```python
from build123d import *

# Parameters (mm, degrees)
F0_W     = 2133.6
F0_H     = 609.6
F1_DEPTH = 762
F3_DEPTH = 15240
F2_W     = 38.1
F2_H     = 152.4
F4_DEPTH = 1270
F2_W_2   = 38.0986694649
F5_DEPTH = 1270
F6_W     = 101.6
F6_H     = 14.6726144286
F6_H_2   = 15.8073855714
F6_H_3   = 15.6187368706
F6_H_4   = 14.8612631294
F7_DEPTH = 12.7


with BuildPart() as f1:
    # F0 (on Top) → F1 (new body)
    with BuildSketch(Plane.XY):
        with Locations((-15.6133426353, -467.8674386665)):
            Rectangle(F0_W, F0_H)
    extrude(amount=F1_DEPTH)

    # F2 (on face) → F3 (cut)
    with BuildSketch(Plane.XZ.offset(772.6674386665)):
        Polygon((-950.7269263268, 152.4), (-950.7269263268, 0), (-15.6133426353, 0), (-15.6133426353, 710.3988881946), (-912.6269263268, 710.3988881946), (-912.6269263268, 152.4), align=None)
        Polygon((881.4002410561, 710.3988881946), (-15.6133426353, 710.3988881946), (-15.6133426353, 0), (919.5002410561, 0), (919.5002410561, 152.4), (881.4002410561, 152.4), align=None)
    extrude(amount=-F3_DEPTH, mode=Mode.SUBTRACT)

    # F2 (on face) → F4 (cut)
    with BuildSketch(Plane.XZ.offset(772.6674386665)):
        Polygon((-950.7269263268, 152.4), (-950.7269263268, 0), (-15.6133426353, 0), (-15.6133426353, 710.3988881946), (-912.6269263268, 710.3988881946), (-912.6269263268, 152.4), align=None)
        with Locations((-1063.3633426353, 76.2)):
            Rectangle(F2_W, F2_H)
        Polygon((-15.6133426353, 710.3988881946), (-15.6133426353, 0), (919.5002410561, 0), (919.5002410561, 152.4), (881.4002410561, 152.4), (881.4002410561, 710.3988881946), align=None)
    extrude(amount=-F4_DEPTH, mode=Mode.SUBTRACT)

    # F2 (on face) → F5 (cut)
    with BuildSketch(Plane.XZ.offset(772.6674386665)):
        with Locations((-1063.3633426353, 76.2)):
            Rectangle(F2_W, F2_H)
        with Locations((1032.1373226322, 76.2)):
            Rectangle(F2_W_2, F2_H)
    extrude(amount=-F5_DEPTH, mode=Mode.SUBTRACT)

    # F6 (on face) → F7 (cut)
    with BuildSketch(Plane.XY.offset(762)):
        with Locations((-682.8922287941, -460.5311314521)):
            Rectangle(F6_W, F6_H)
        with Locations((-682.8922287941, -475.7711314521)):
            Rectangle(F6_W, F6_H_2)
        with Locations((-276.6795860052, -475.6768071018)):
            Rectangle(F6_W, F6_H_3)
        with Locations((-276.6795860052, -460.4368071018)):
            Rectangle(F6_W, F6_H_4)
        with Locations((245.4529007345, -475.6768071018)):
            Rectangle(F6_W, F6_H_3)
        with Locations((245.4529007345, -460.4368071018)):
            Rectangle(F6_W, F6_H_4)
        with Locations((651.6655435234, -475.7711314521)):
            Rectangle(F6_W, F6_H_2)
        with Locations((651.6655435234, -460.5311314521)):
            Rectangle(F6_W, F6_H)
    extrude(amount=-F7_DEPTH, mode=Mode.SUBTRACT)


solid = f1.part
```
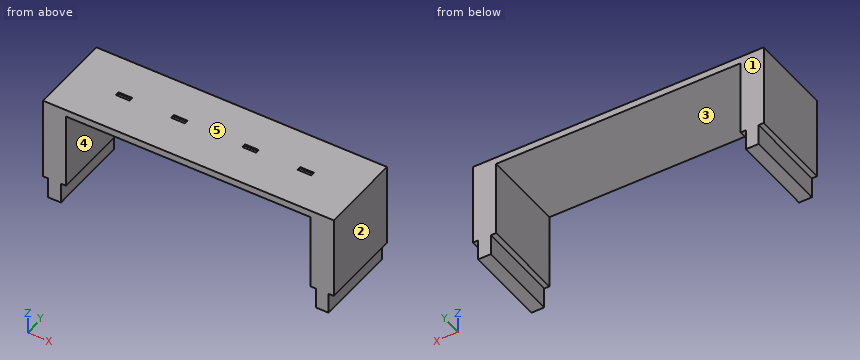
Source: CAD feature listing. Evaluate the final solid. Frame: model axes, mm. Face numbers are marked on the shaded views. A direction names the side the tool comes from. Round coordinates to 2 decimals unless told otherwise and drop trailing zeros. Order: outer loops, then holes, each group sorted by start corner. A loop starts at its lowest first (then second) coordinate and runs counter-clockwise, first axis right, second up. Notation, with made-up numbers: (-15, -28) -> (25, -28) arc R29 ccw to (25, -3) -> close; hole circle Ø5 at (55, 70.25). An arc over 180 degrees is marked (long way). One line per item, written item: value. Start each with the question number.
Q1. Draft query along X for the marked faces 1, 2 and 3. Return one class per face: pulls with the +X half, pulls with the -X half, needs draft (parallel to the pull), parting line crosses it, or undercut.
Q2. Material intervals for probe 1 along X at (y, z) = (-463.5, 530); probe 2 along X at (y, z) = (-246, 99); probe 3 along Z at (x, y) = (413, -530.5), sorted ascending.
Q3. Section query B-B (y = -647). Return the cut outline in (x, z).
Q4. Section query D-D (x = 339). Return the cut outline in (y, z).
Q5. Section query A-A (z = 615). Return the cut outline in (x, y).
Q6. Section query C-C (z = 123). Return the cut outline in (x, y), plus the area to 3 significant figures.
Q7. Pin query (flat end, axial travel): pin 1 (5 mm diameter, centred on x = -188, y = -357, fed in from -Z); pin 2 (8 mm diameter, centred on y = -229.5, z = 122.5, fed in from -X); pin 3 (15 mm diameter, centred on x = -292.5, y = -463.5, fed in from +Z). Return the tip coordinate at first contact, or that it passes through.
Q8. Access query for the marked faces 4 and 5. Directions: +Z, -Z, +X, -X, +Y, -Y. A direction counts if a zero-diameter tool reaches every point of the face in a straight line with its end or side. Return the directions, or none.
Findings below:
1. face 1: needs draft
1. face 2: pulls with the +X half
1. face 3: undercut
2. probe 1: -1082.41 to -912.63, 881.4 to 1051.19
2. probe 2: -1044.31 to -950.73, 919.5 to 1013.09
2. probe 3: 710.4 to 762
3. outline: (-1082.41, 152.4) -> (-1044.31, 152.4) -> (-1044.31, 0) -> (-950.73, 0) -> (-950.73, 152.4) -> (-912.63, 152.4) -> (-912.63, 710.4) -> (881.4, 710.4) -> (881.4, 152.4) -> (919.5, 152.4) -> (919.5, 0) -> (1013.09, 0) -> (1013.09, 152.4) -> (1051.19, 152.4) -> (1051.19, 762) -> (-1082.41, 762) -> close
4. outline: (-772.67, 710.4) -> (-163.07, 710.4) -> (-163.07, 762) -> (-772.67, 762) -> close
5. outline: (-1082.41, -772.67) -> (-912.63, -772.67) -> (-912.63, -163.07) -> (-1082.41, -163.07) -> close; (881.4, -772.67) -> (1051.19, -772.67) -> (1051.19, -163.07) -> (881.4, -163.07) -> close
6. outline: (-1044.31, -772.67) -> (-950.73, -772.67) -> (-950.73, -163.07) -> (-1044.31, -163.07) -> close; (919.5, -772.67) -> (1013.09, -772.67) -> (1013.09, -163.07) -> (919.5, -163.07) -> close
6. area: 114,000 mm²
7. pin 1: z = 710.4
7. pin 2: x = -1044.31
7. pin 3: z = 749.3
8. face 4: -Z, +Y, -Y
8. face 5: +Z, +X, -X, +Y, -Y
